Can you work these out from the model? Positions are in its coordinate system, mm. A direction names the side the tool comes from. Coordinates: 2 decimals unless noted, no trailing zeros. Order: outer loops, then holes, each group sorted by start corner. A loop starts at its lowest first (then second) coordinate and runs counter-clockwise, first axis right, second up. Notation, with made-up numbers: (54.5, 88.25) - (95.5, 88.25) arc R16 cw to (95.5, 117.25) - close; hole circle Ø9 at (74, 35.5). An arc over 180 degrees is marked (long way). Return JSON: item names as keys, results as strings. Group by question number.
1) For pin 1 Ø1.7 at (y, z) = (-2.5, 9) entering from -X; pin 2 Ø2 at (x, y) = (-13.5, -4.5) entering from +Z; pin 3 Ø1 at (y, z) = (0.5, 3.5) entering from -X, each with a flat end and sliding along its axis, tell me the tip position at first contact or that it passes through.
2) Imagine slicing it at B-B (x = -19). Write out the boundary of the cut face in (y, z).
3) If I drill on line 1 along X through (y, z) = (-6.25, 6); line 2 along Y through (x, z) = (-13, 5); line 3 along X through (y, z) = (-2.25, 8.5), over which ranges is the centre line in solid material (lowest first)?
4) Which directions (+Z, -Z, +X, -X, +Y, -Y) give clear straight access to the entire face, cutting with the end or side of a thin tool? Please do faces 1 (the face through (-13.1, -2, 9)), 2 (the face through (-14.64, -1.85, 3.57)), 3 (the face through (-5.1, -2, 7)).
5) Imagine slicing it at A-A (y = -2.5). Write out the boundary of the cut face in (x, z).
6) Imagine slicing it at C-C (x = -7). Write out the boundary of the cut face in (y, z), and give its area (3 significant figures).
```python
from build123d import *

# Parameters (mm, degrees)
SKETCH001_R  = 4.5
PAD001_DEPTH = 5
SKETCH002_R  = 3
PAD002_DEPTH = 10
SKETCH003_W  = 9
SKETCH003_H  = 3
POCKET_DEPTH = 7
CHAMFER_SIZE = 0.8


with BuildPart() as part:
    # Sketch001 (on Face1 of ShapeBinder) → Pad001 (new body)
    with BuildSketch(Plane(origin=(-5.1, 0, 0), x_dir=(0, -1, 0), z_dir=(-1, 0, 0))):
        with Locations((2.5, 6.5)):
            Circle(SKETCH001_R)
    extrude(amount=PAD001_DEPTH)

    # Sketch002 (on Face3 of Pad001) → Pad002 (join)
    with BuildSketch(Plane(origin=(-10.1, 0, 0), x_dir=(0, -1, 0), z_dir=(-1, 0, 0))):
        with Locations((2.5, 6.5)):
            Circle(SKETCH002_R)
    extrude(amount=PAD002_DEPTH)

    # Sketch003 (on Face5 of Pad002) → Pocket (cut)
    with BuildSketch(Plane(origin=(-20.1, 0, 0), x_dir=(0, -1, 0), z_dir=(-1, 0, 0))):
        with Locations((2.5, 9.5)):
            Rectangle(SKETCH003_W, SKETCH003_H)
    extrude(amount=-POCKET_DEPTH, mode=Mode.SUBTRACT)

    # Chamfer
    chamfer_edges = [part.edges().sort_by_distance(p)[0] for p in [
        (-20.1, -5.397777, 7.276457),
        (-20.1, -2.5, 8),
        (-20.1, -1.723543, 3.602223),
    ]]
    chamfer(chamfer_edges, length=CHAMFER_SIZE)


solid = part.part
```
Calculated:
{
 "1": {"pin 1": "x = -13.1", "pin 2": "z = 9.3", "pin 3": "x = -10.1"},
 "2": {"outline": "(-5.1, 8) arc R3 ccw (long way) to (0.1, 8) - close"},
 "3": {"line 1": "-10.1 to -5.1", "line 2": "-5.1 to 0.1", "line 3": "-13.1 to -5.1"},
 "4": {"face 1": "+Z, -X, +Y, -Y", "face 2": "-X", "face 3": "+Z, -Z, +X, +Y, -Y"},
 "5": {"outline": "(-20.1, 4.3) - (-19.3, 3.5) - (-10.1, 3.5) - (-10.1, 2) - (-5.1, 2) - (-5.1, 11) - (-10.1, 11) - (-10.1, 9.5) - (-13.1, 9.5) - (-13.1, 8) - (-19.3, 8) - (-20.1, 7.2) - close"},
 "6": {"outline": "circle Ø9 at (-2.5, 6.5)", "area": "63.6 mm2"}
}
